```python
from build123d import *

# Parameters (mm, degrees)
DODANIE_WYCI_GNI_CIE1_DEPTH      = 13.5
DODANIE_WYCI_GNI_CIE1_DEPTH_BACK = 13.5
SZKIC1_W                         = 222
SZKIC1_H                         = 125
SZKIC1_R                         = 13
SZKIC1_R_2                       = 4
SZKIC4_W                         = 15
SZKIC4_H                         = 27
DODANIE_WYCI_GNI_CIE4_DEPTH      = 36
SZKIC13_R                        = 38.75
WYTNIJ_WYCI_GNI_CIE4_DEPTH       = 17
SZKIC15_R                        = 44.5
WYTNIJ_WYCI_GNI_CIE5_DEPTH       = 5
POCHYLENIE1_ANGLE                = 45
DODANIE_WYCI_GNI_CIE6_START      = 21
SZKIC16_R                        = 13
SZKIC16_R_2                      = 4
DODANIE_WYCI_GNI_CIE6_DEPTH      = 21
SZKIC5_R                         = 6
WYTNIJ_WYCI_GNI_CIE3_DEPTH       = 246.308988828
WYTNIJ_WYCI_GNI_CIE6_DEPTH       = 156.971952607
ZAOKR_GLENIE1_R                  = 30
ZAOKR_GLENIE2_R                  = 30
SZKIC19_W                        = 40
SZKIC19_H                        = 60
DODANIE_WYCI_GNI_CIE7_DEPTH      = 48
WYTNIJ_WYCI_GNI_CIE7_REACH       = 184.64
SZKIC23_R                        = 20
WYTNIJ_WYCI_GNI_CIE8_REACH       = 174.137
ZAOKR_GLENIE4_R                  = 5
ZAOKR_GLENIE5_R                  = 5
WYTNIJ_WYCI_GNI_CIE9_DEPTH       = 48


with BuildPart() as part:
    # Szkic1 → Dodanie-wyciągnięcie1 (new, two sides: drawn at the far end of the back side and taken through both)
    with BuildSketch(Plane.XY.offset(-DODANIE_WYCI_GNI_CIE1_DEPTH_BACK)):
        Rectangle(SZKIC1_W, SZKIC1_H)
        Circle(SZKIC1_R, mode=Mode.SUBTRACT)
        with Locations((-32, 0)):
            Circle(SZKIC1_R_2, mode=Mode.SUBTRACT)
        with Locations((-16, 27.712812921)):
            Circle(SZKIC1_R_2, mode=Mode.SUBTRACT)
        with Locations((16, 27.712812921)):
            Circle(SZKIC1_R_2, mode=Mode.SUBTRACT)
        with Locations((32, 0)):
            Circle(SZKIC1_R_2, mode=Mode.SUBTRACT)
        with Locations((16, -27.712812921)):
            Circle(SZKIC1_R_2, mode=Mode.SUBTRACT)
        with Locations((-16, -27.712812921)):
            Circle(SZKIC1_R_2, mode=Mode.SUBTRACT)
    extrude(amount=DODANIE_WYCI_GNI_CIE1_DEPTH + DODANIE_WYCI_GNI_CIE1_DEPTH_BACK)

    # Szkic4 → Dodanie-wyciągnięcie4 (add)
    with BuildSketch(Plane(origin=(0, 62.5, 0), x_dir=(1, 0, 0), z_dir=(0, 1, 0))):
        with Locations((-103.5, 0)):
            Rectangle(SZKIC4_W, SZKIC4_H)
        with Locations((-53.5, 0)):
            Rectangle(SZKIC4_W, SZKIC4_H)
        with Locations((53.5, 0)):
            Rectangle(SZKIC4_W, SZKIC4_H)
        with Locations((103.5, 0)):
            Rectangle(SZKIC4_W, SZKIC4_H)
    extrude(amount=DODANIE_WYCI_GNI_CIE4_DEPTH)

    # Szkic13 → Wytnij-wyciągnięcie4 (cut)
    with BuildSketch(Plane.XY.offset(13.5)):
        Circle(SZKIC13_R)
    extrude(amount=-WYTNIJ_WYCI_GNI_CIE4_DEPTH, mode=Mode.SUBTRACT)

    # Szkic15 → Wytnij-wyciągnięcie5 (cut)
    with BuildSketch(Plane.XY.offset(13.5)):
        Circle(SZKIC15_R)
    extrude(amount=-WYTNIJ_WYCI_GNI_CIE5_DEPTH, mode=Mode.SUBTRACT)

    # Pochylenie1
    pochylenie1_faces = [part.faces().sort_by_distance(p)[0] for p in [
        (-44.5, 0, 11),
    ]]
    draft(pochylenie1_faces, Plane.XY.offset(8.5), POCHYLENIE1_ANGLE)

    # Szkic16 → Dodanie-wyciągnięcie6 (add)
    with BuildSketch(Plane(origin=(0, 0, -13.5), x_dir=(-1, 0, 0), z_dir=(0, 0, -1)).offset(DODANIE_WYCI_GNI_CIE6_START)):
        Polygon((-111, 98.5), (-111, -62.5), (111, -62.5), (111, 98.5), (96, 98.5), (96, 62.5), (61, 62.5), (61, 98.5), (46, 98.5), (46, 62.5), (-46, 62.5), (-46, 98.5), (-61, 98.5), (-61, 62.5), (-96, 62.5), (-96, 98.5), align=None)
        with Locations(Location((0, 0, 0), (0, 0, 180))):
            Circle(SZKIC16_R, mode=Mode.SUBTRACT)
        with Locations(Location((32, 0, 0), (0, 0, 180))):
            Circle(SZKIC16_R_2, mode=Mode.SUBTRACT)
        with Locations(Location((16, 27.712812921, 0), (0, 0, 180))):
            Circle(SZKIC16_R_2, mode=Mode.SUBTRACT)
        with Locations(Location((-16, 27.712812921, 0), (0, 0, 180))):
            Circle(SZKIC16_R_2, mode=Mode.SUBTRACT)
        with Locations(Location((-32, 0, 0), (0, 0, 180))):
            Circle(SZKIC16_R_2, mode=Mode.SUBTRACT)
        with Locations(Location((-16, -27.712812921, 0), (0, 0, 180))):
            Circle(SZKIC16_R_2, mode=Mode.SUBTRACT)
        with Locations(Location((16, -27.712812921, 0), (0, 0, 180))):
            Circle(SZKIC16_R_2, mode=Mode.SUBTRACT)
    extrude(amount=-DODANIE_WYCI_GNI_CIE6_DEPTH)

    # Szkic5 → Wytnij-wyciągnięcie3 (cut, through all)
    with BuildSketch(Plane.ZY.offset(111)):
        with Locations((-10.5, 78.5)):
            Circle(SZKIC5_R)
    extrude(amount=-WYTNIJ_WYCI_GNI_CIE3_DEPTH, mode=Mode.SUBTRACT)

    # Szkic18 → Wytnij-wyciągnięcie6 (cut, through all)
    with BuildSketch(Plane(origin=(0, 0, -34.5), x_dir=(-1, 0, 0), z_dir=(0, 0, -1))):
        Polygon((111, 22.5), (46, -62.5), (111, -62.5), align=None)
        Polygon((-111, -62.5), (-46, -62.5), (-111, 22.5), align=None)
    extrude(amount=-WYTNIJ_WYCI_GNI_CIE6_DEPTH, mode=Mode.SUBTRACT)

    # Zaokrąglenie1
    zaokr_glenie1_edges = [part.edges().sort_by_distance(p)[0] for p in [
        (-111, 22.5, -10.5),
    ]]
    fillet(zaokr_glenie1_edges, radius=ZAOKR_GLENIE1_R)

    # Zaokrąglenie2
    zaokr_glenie2_edges = [part.edges().sort_by_distance(p)[0] for p in [
        (-46, -62.5, -10.5),
        (111, 22.5, -10.5),
        (46, -62.5, -10.5),
    ]]
    fillet(zaokr_glenie2_edges, radius=ZAOKR_GLENIE2_R)

    # Szkic19 → Dodanie-wyciągnięcie7 (add)
    with BuildSketch(Plane(origin=(0, 0, -34.5), x_dir=(-1, 0, 0), z_dir=(0, 0, -1))):
        with Locations((0, -92.5)):
            Rectangle(SZKIC19_W, SZKIC19_H)
    extrude(amount=-DODANIE_WYCI_GNI_CIE7_DEPTH)

    # Szkic23 → Wytnij-wyciągnięcie7 (cut, up to next)
    with BuildSketch(Plane(origin=(20, 0, 0), x_dir=(0, 0, -1), z_dir=(1, 0, 0)), mode=Mode.PRIVATE) as wytnij_wyci_gni_cie7_sk1:
        with Locations(Location((10.5, -92.5, 0), (0, 0, 90))):
            Circle(SZKIC23_R)
    wytnij_wyci_gni_cie7_tool1 = extrude(wytnij_wyci_gni_cie7_sk1.sketch, amount=-WYTNIJ_WYCI_GNI_CIE7_REACH, mode=Mode.PRIVATE) & part.part
    add(wytnij_wyci_gni_cie7_tool1.solids().sort_by_distance((20, -92.5, -10.5))[0], mode=Mode.SUBTRACT)

    # Szkic24 → Wytnij-wyciągnięcie8 (cut, up to next)
    with BuildSketch(Plane(origin=(0, 0, -34.5), x_dir=(-1, 0, 0), z_dir=(0, 0, -1)), mode=Mode.PRIVATE) as wytnij_wyci_gni_cie8_sk1:
        with BuildLine():
            Line((-96, 62.5), (-61, 62.5))
            ThreePointArc((-61, 62.5), (-78.5, 45), (-96, 62.5))
        make_face()
    wytnij_wyci_gni_cie8_tool1 = extrude(wytnij_wyci_gni_cie8_sk1.sketch, amount=-WYTNIJ_WYCI_GNI_CIE8_REACH, mode=Mode.PRIVATE) & part.part
    # Szkic24 → Wytnij-wyciągnięcie8 (cut, up to next)
    with BuildSketch(Plane(origin=(0, 0, -34.5), x_dir=(-1, 0, 0), z_dir=(0, 0, -1)), mode=Mode.PRIVATE) as wytnij_wyci_gni_cie8_sk2:
        with BuildLine():
            Line((61, 62.5), (96, 62.5))
            ThreePointArc((96, 62.5), (78.5, 45), (61, 62.5))
        make_face()
    wytnij_wyci_gni_cie8_tool2 = extrude(wytnij_wyci_gni_cie8_sk2.sketch, amount=-WYTNIJ_WYCI_GNI_CIE8_REACH, mode=Mode.PRIVATE) & part.part
    add(wytnij_wyci_gni_cie8_tool1.solids().sort_by_distance((78.5, 55.072769, -34.5))[0], mode=Mode.SUBTRACT)
    add(wytnij_wyci_gni_cie8_tool2.solids().sort_by_distance((-78.5, 55.072769, -34.5))[0], mode=Mode.SUBTRACT)

    # Zaokrąglenie4
    zaokr_glenie4_edges = [part.edges().sort_by_distance(p)[0] for p in [
        (20, -62.5, -10.5),
        (-20, -62.5, -10.5),
    ]]
    fillet(zaokr_glenie4_edges, radius=ZAOKR_GLENIE4_R)

    # Zaokrąglenie5
    zaokr_glenie5_edges = [part.edges().sort_by_distance(p)[0] for p in [
        (0, -122.5, -34.5),
        (0, -122.5, 13.5),
    ]]
    fillet(zaokr_glenie5_edges, radius=ZAOKR_GLENIE5_R)

    # Szkic25 → Wytnij-wyciągnięcie9 (cut)
    with BuildSketch(Plane.XY.offset(13.5)):
        with BuildLine():
            Line((-60.951491344, -10.353512592), (-74.069286372, 21.36621852))
            ThreePointArc((-74.069286372, 21.36621852), (-84.742802137, 24.999340902), (-86.957683747, 13.944124193))
            Line((-86.957683747, 13.944124193), (-66.106850294, -13.322350323))
            ThreePointArc((-66.106850294, -13.322350323), (-62.22665594, -14.099736361), (-60.951491344, -10.353512592))
        make_face()
        with BuildLine():
            Line((66.106850294, -13.322350323), (86.957683747, 13.944124193))
            ThreePointArc((86.957683747, 13.944124193), (84.742802137, 24.999340902), (74.069286372, 21.36621852))
            Line((74.069286372, 21.36621852), (60.951491344, -10.353512592))
            ThreePointArc((60.951491344, -10.353512592), (62.22665594, -14.099736361), (66.106850294, -13.322350323))
        make_face()
    extrude(amount=-WYTNIJ_WYCI_GNI_CIE9_DEPTH, mode=Mode.SUBTRACT)


solid = part.part
```
Read the model definition and answer for the solid it produces. Units are mm, in the model's axes. A direction names the side the tool comes from. Give positions to 0.01 mm unless a question says otherwise; leave off trailing zeros. Write each loop counter-clockwise with the first axis right and the second up, starting at its lowest first coordinate (ties: lowest second). Pieces come first, ordered by that corner, then holes. Notation, with made-up numbers: (-13, 37) -> (-1, 37) arc R25 ccw to (-1, 52) -> close; hole circle Ø4 at (-27.5, 54.25). An arc over 180 degrees is marked (long way). Answer as a JSON object with one key per item and string values.
1) Section B-B on y = -99 is taken. Write down the section's boundary in (x, z), then the cut area to 3 significant figures.
Findings below:
{"outline": "(-20, -34.5) -> (20, -34.5) -> (20, -29.41) -> (-20, -29.41) -> close; (-20, 8.41) -> (20, 8.41) -> (20, 13.5) -> (-20, 13.5) -> close", "area": "407 mm^2"}
2) Section C-C on x = -78.5 is taken. Write down the section's boundary in (y, z), then the cut area to 3 significant figures.
Findings below:
{"outline": "(-20, -34.5) -> (2.88, -34.5) -> (2.88, 13.5) -> (-20, 13.5) -> close; (25.57, -34.5) -> (45, -34.5) -> (45, 13.5) -> (25.57, 13.5) -> close", "area": "2,030 mm^2"}
3) Section A-A on x = 0 is taken. Write down the section's boundary in (y, z), then the cut area to 3 significant figures.
Findings below:
{"outline": "(-122.5, -29.5) arc R5 ccw to (-117.5, -34.5) -> (-13, -34.5) -> (-13, -3.5) -> (-38.75, -3.5) -> (-38.75, 8.5) -> (-44.5, 8.5) -> (-49.5, 13.5) -> (-117.5, 13.5) arc R5 ccw to (-122.5, 8.5) -> close; (13, -34.5) -> (62.5, -34.5) -> (62.5, 13.5) -> (49.5, 13.5) -> (44.5, 8.5) -> (38.75, 8.5) -> (38.75, -3.5) -> (13, -3.5) -> close; hole circle Ø40 at (-92.5, -10.5)", "area": "5,410 mm^2"}
4) Flat-ended cylindrical pins translate along their axes: pin 1 Ø8 at (y, z) = (-32.5, 7.5) entering from +X; pin 2 Ø6 at (x, z) = (-34, 5) entering from +Y; pin 3 Ø8 at (x, y) = (41.5, 72.5) entering from +Z; pin 4 Ø4 at (y, z) = (-11.5, -20.5) entering from -X. Find the tip coordinate at first contact, or state that the pin passes through.
Findings below:
{"pin 1": "stops at x = 72", "pin 2": "stops at y = 62.5", "pin 3": "passes through", "pin 4": "stops at x = -86.53"}
5) Section D-D on z = -26 is taken. Count the separate pieces of the cut face and the enclosed holes in it, then the cut area to 3 significant figures.
Findings below:
{"separate pieces": "2", "enclosed holes": "9", "area": "23,000 mm^2"}
6) For a pull along Z with two mould halves and no side action, classify faces 1 (the cylindrical face through (-103.6, 84.45, -11.28)), 2 (the flat face through (-76.678, 0.502, -10.164)) as pulls with the +Z half, pulls with the -Z half, needs draft (parallel to the pull), parting line crosses it, or undercut.
Findings below:
{"face 1": "undercut", "face 2": "needs draft"}
7) A tool of negligible diameter and unlimited length cuts with its end or side. For faces 3 (the flat face through (67.602, 5.728, -10.164)), 4 (the flat face through (96, 84, -16)), 5 (the flat face through (-20, -114, -11)), 6 (the flat face through (-111, 65, -11)), from which of +Z, -Z, +X, -X, +Y, -Y can it reach the whole face along a straight path? Write none if from no direction.
Findings below:
{"face 3": "+Z, -Z", "face 4": "+Z, -Z, +Y", "face 5": "+Z, -Z, -X, -Y", "face 6": "+Z, -Z, -X, +Y, -Y"}
8) Straight lines are drawn through the part: probe 1 along X at (y, z) = (72, -16); probe 2 along X at (y, z) = (-24.5, -12); probe 3 along X at (y, z) = (-29.5, -13.5). For each, find the intervals that lie inside material, in ascending order. Write a range as from..to.
Findings below:
{"probe 1": "x = -111..-96, -61..-46, 46..61, 96..111", "probe 2": "x = -75.06..-18.38, -13.62..13.62, 18.38..75.06", "probe 3": "x = -71.24..-19.58, -12.42..12.42, 19.58..71.24"}
